```python
from build123d import *

# Parameters (mm, degrees)
BOSS_EXTRUDE3_DEPTH = 2
BOSS_EXTRUDE4_DEPTH = 7
FILLET2_R           = 1


with BuildPart() as part:
    # Sketch1 → Boss-Extrude3 (new body)
    with BuildSketch(Plane.XY):
        with BuildLine():
            Line((-5, 15.1), (-5, 0.9))
            Line((-5, 0.9), (-5, -1.1))
            Line((-5, -1.1), (-5, -15.1))
            Line((-5, -15.1), (-6, -15.1))
            ThreePointArc((-6, -15.1), (-7, -16.1), (-6, -17.1))
            Line((-6, -17.1), (5, -17.1))
            Line((5, -17.1), (6, -17.1))
            ThreePointArc((6, -17.1), (7, -16.1), (6, -15.1))
            Line((6, -15.1), (5, -15.1))
            Line((5, -15.1), (5, -1.1))
            Line((5, -1.1), (5, 0.9))
            Line((5, 0.9), (5, 15.1))
            Line((5, 15.1), (6, 15.1))
            ThreePointArc((6, 15.1), (7, 16.1), (6, 17.1))
            Line((6, 17.1), (5, 17.1))
            Line((5, 17.1), (-5, 17.1))
            Line((-5, 17.1), (-6, 17.1))
            ThreePointArc((-6, 17.1), (-7, 16.1), (-6, 15.1))
            Line((-6, 15.1), (-5, 15.1))
        make_face()
    extrude(amount=BOSS_EXTRUDE3_DEPTH)

    # Sketch3 → Boss-Extrude4 (add)
    with BuildSketch(Plane.XY.offset(2)):
        with BuildLine():
            Line((-6, 15.1), (-5, 15.1))
            Line((-5, 15.1), (5, 15.1))
            Line((5, 15.1), (6, 15.1))
            ThreePointArc((6, 15.1), (7, 16.1), (6, 17.1))
            Line((6, 17.1), (-6, 17.1))
            ThreePointArc((-6, 17.1), (-7, 16.1), (-6, 15.1))
        make_face()
        with BuildLine():
            Line((-6, -15.1), (-5, -15.1))
            Line((-5, -15.1), (5, -15.1))
            Line((5, -15.1), (6, -15.1))
            ThreePointArc((6, -15.1), (7, -16.1), (6, -17.1))
            Line((6, -17.1), (-6, -17.1))
            ThreePointArc((-6, -17.1), (-7, -16.1), (-6, -15.1))
        make_face()
    extrude(amount=BOSS_EXTRUDE4_DEPTH)

    # Fillet2
    fillet2_edges = [part.edges().sort_by_distance(p)[0] for p in [
        (-5, 15.1, 1),
        (-5, -15.1, 1),
        (5, 15.1, 1),
        (5, -15.1, 1),
    ]]
    fillet(fillet2_edges, radius=FILLET2_R - 0.0001)  # a hair under: the kernel refuses the full size


solid = part.part
```
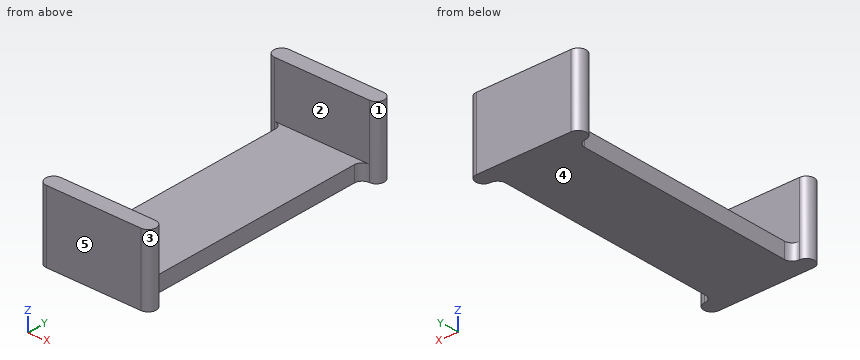
CAD build for the part. Positions are in the model's coordinates, mm. Face numbers are marked on the shaded views. A direction names the side the tool comes from. Give positions to 0.01 mm unless a question says otherwise; leave off trailing zeros. Write each loop counter-clockwise with the first axis right and the second up, starting at its lowest first coordinate (ties: lowest second). Pieces come first, ordered by that corner, then holes. Notation, with made-up numbers: M -21.5,-7 L 20.5,-7 A26 cw 20.5,28 Z; hole C 71.25,-10 d10. An arc over 180 degrees is marked long. Return JSON: item names as keys, results as strings. Group by question number.
(1) 3-axis set-ups, long thin cutter, end or side, ignore diameter. For the marked faces 1 and 2: which of +Z, -Z, +X, -X, +Y, -Y reach the whole face in a straight line?
(2) Drill centre lines: L1, parallel to Y at x = 3.25, z = 4.25; L2, parallel to Y at x = 6.75, z = 4.5; L3, parallel to Z at x = 4.75, y = 12. Where is each one in solid material? Low to high. Write a range as [from, to].
(3) Band-saw the part on A-A (z = 6.5). Give the cut face in (x, y).
(4) Flat gauge pins, fed straight in: pin 1 Ø6 at (x, y) = (-1, -9.5) entering from -Z; pin 2 Ø1 at (y, z) = (-7, 0.5) entering from +X; pin 3 Ø6 at (x, y) = (1, 0) entering from +Z; pin 4 Ø1.6 at (y, z) = (-1, 1) entering from -X. Where does each tip first touch, or does it go through?
(5) Mould opens along Y. For the marked faces 3, 4 and 5 say: pulls with the +Y half, pulls with the -Y half, needs draft (parallel to the pull), parting line crosses it, or undercut.
(6) Band-saw the part on B-B (x = -0.75). Give the cut face in (y, z), and give its area (3 significant figures).
(7) Band-saw the part on C-C (y = -7). Give the cut face in (x, z), and give its area (3 significant figures).
Entries:
{
 "1": {"face 1": "+Z, -Z, +X", "face 2": "+Z, +X, -X"},
 "2": {"L1": "y = [-17.1, -15.1], [15.1, 17.1]", "L2": "y = [-16.76, -15.44], [15.44, 16.76]", "L3": "z = [0, 2]"},
 "3": {"outline": "M -6,-17.1 L 6,-17.1 A1 ccw 6,-15.1 L -6,-15.1 A1 ccw Z; M -6,15.1 L 6,15.1 A1 ccw 6,17.1 L -6,17.1 A1 ccw Z"},
 "4": {"pin 1": "stops at z = 0", "pin 2": "stops at x = 5", "pin 3": "stops at z = 2", "pin 4": "stops at x = -5"},
 "5": {"face 3": "undercut", "face 4": "needs draft", "face 5": "pulls with the -Y half"},
 "6": {"outline": "M -17.1,0 L 17.1,0 L 17.1,9 L 15.1,9 L 15.1,2 L -15.1,2 L -15.1,9 L -17.1,9 Z", "area": "96.4 mm^2"},
 "7": {"outline": "M -5,0 L 5,0 L 5,2 L -5,2 Z", "area": "20.0 mm^2"}
}
